```python
from build123d import *

# Parameters (mm, degrees)
SKETCH1_R           = 13.1
SKETCH1_R_2         = 1.75
BOSS_EXTRUDE1_DEPTH = 7
SKETCH2_R           = 13.1
SKETCH2_R_2         = 11
BOSS_EXTRUDE2_DEPTH = 2
SKETCH3_W           = 60
SKETCH3_H           = 16
SKETCH3_R           = 1.75
BOSS_EXTRUDE3_DEPTH = 4
SKETCH4_R           = 3.75
CUT_EXTRUDE1_DEPTH  = 4


with BuildPart() as part:
    # Sketch1 → Boss-Extrude1 (new body)
    with BuildSketch(Plane.XY):
        with BuildLine():
            Line((-30, -55), (30, -55))
            Line((30, -55), (30, -39))
            Line((30, -39), (24.811961667, 3.060483334))
            ThreePointArc((24.811961667, 3.060483334), (0, 25), (-24.811961667, 3.060483334))
            Line((-24.811961667, 3.060483334), (-30, -39))
            Line((-30, -39), (-30, -55))
        make_face()
        Circle(SKETCH1_R, mode=Mode.SUBTRACT)
        with Locations((-20, -47)):
            Circle(SKETCH1_R_2, mode=Mode.SUBTRACT)
        with Locations((20, -47)):
            Circle(SKETCH1_R_2, mode=Mode.SUBTRACT)
    extrude(amount=BOSS_EXTRUDE1_DEPTH)

    # Sketch2 → Boss-Extrude2 (add)
    with BuildSketch(Plane.XY.offset(7)):
        Circle(SKETCH2_R)
        Circle(SKETCH2_R_2, mode=Mode.SUBTRACT)
    extrude(amount=-BOSS_EXTRUDE2_DEPTH)

    # Sketch3 → Boss-Extrude3 (add)
    with BuildSketch(Plane.XY.offset(7)):
        with Locations((0, -47)):
            Rectangle(SKETCH3_W, SKETCH3_H)
        with Locations((20, -47)):
            Circle(SKETCH3_R, mode=Mode.SUBTRACT)
        with Locations((-20, -47)):
            Circle(SKETCH3_R, mode=Mode.SUBTRACT)
    extrude(amount=BOSS_EXTRUDE3_DEPTH)

    # Sketch4 → Cut-Extrude1 (cut)
    with BuildSketch(Plane(origin=(0, 0, 0), x_dir=(-1, 0, 0), z_dir=(0, 0, -1))):
        with Locations((-20, -47)):
            Circle(SKETCH4_R)
        with Locations((20, -47)):
            Circle(SKETCH4_R)
    extrude(amount=-CUT_EXTRUDE1_DEPTH, mode=Mode.SUBTRACT)


solid = part.part
```
Verification items for the finished model (mm, model axes). A direction names the side the tool comes from. Round coordinates to 2 decimals unless told otherwise and drop trailing zeros. Order: outer loops, then holes, each group sorted by start corner. A loop starts at its lowest first (then second) coordinate and runs counter-clockwise, first axis right, second up.
1) Draft check along X on faces 1 (the flat face through (30, -47, 5)), 2 (the flat face through (-21, -49, 4)), 3 (the flat face through (-27.37, -17.68, 3.45)). Enter one of: +X half, -X half, draft (parallel to the pull), parting line (faces both ways), or undercut.
Geometry says:
face 1: +X half
face 2: undercut
face 3: -X half
2) Cross-section at B-B, the plane x = 0. Record the cut outline in (y, z).
Geometry says:
outline: (-55, 0) - (-13.1, 0) - (-13.1, 5) - (-11, 5) - (-11, 7) - (-39, 7) - (-39, 11) - (-55, 11) - close; (11, 5) - (13.1, 5) - (13.1, 0) - (25, 0) - (25, 7) - (11, 7) - close
3) Cross-section at A-A, the plane z = 2.5. Record the cut outline in (x, y), plus the area to 3 significant figures.
Geometry says:
outline: (-30, -55) - (30, -55) - (30, -39) - (24.81, 3.06) arc R25 ccw to (-24.81, 3.06) - (-30, -39) - close; hole circle Ø7.5 at (-20, -47); hole circle Ø26.2 at (0, 0); hole circle Ø7.5 at (20, -47)
area: 3,470 mm2
4) Tool access check on faces 4 (the flat face through (0, -14, 7)), 5 (the flat face through (-30, -47, 5)), 6 (the flat face through (19, -49, 4)). Record the directions out of +Z, -Z, +X, -X, +Y, -Y that give a thin tool (end or side, any length) a straight path to the whole face; none if there is none.
Geometry says:
face 4: +Z, +X, -X, +Y
face 5: +Z, -Z, -X, +Y, -Y
face 6: -Z
5) Cross-section at C-C, the plane y = -47. Record the cut outline in (x, z), plus the area to 3 significant figures.
Geometry says:
outline: (-30, 0) - (-23.75, 0) - (-23.75, 4) - (-21.75, 4) - (-21.75, 11) - (-30, 11) - close; (-18.25, 4) - (-16.25, 4) - (-16.25, 0) - (16.25, 0) - (16.25, 4) - (18.25, 4) - (18.25, 11) - (-18.25, 11) - close; (21.75, 4) - (23.75, 4) - (23.75, 0) - (30, 0) - (30, 11) - (21.75, 11) - close
area: 551 mm2
6) Material ranges on line 1 (X direction, y = -47, z = 5.75); line 2 (Y direction, x = 20, z = 7.5); line 3 (Y direction, x = 0, z = 6.1), recorded low to high.
Geometry says:
line 1: x = -30 to -21.75, -18.25 to 18.25, 21.75 to 30
line 2: y = -55 to -48.75, -45.25 to -39
line 3: y = -55 to -11, 11 to 25
7) Cross-section at D-D, the plane z = 9. Record the cut outline in (x, y), plus the area to 3 significant figures.
Geometry says:
outline: (-30, -55) - (30, -55) - (30, -39) - (-30, -39) - close; hole circle Ø3.5 at (-20, -47); hole circle Ø3.5 at (20, -47)
area: 941 mm2
8) Depth check by flat-ended pin: pin 1 (8 mm diameter, centred on x = -3.5, y = 1, fed in from -Z); pin 2 (6 mm diameter, centred on x = 13, y = -27.5, fed in from -Z); pin 3 (4.5 mm diameter, centred on x = 20, y = -47, fed in from -Z); pin 4 (1 mm diameter, centred on x = -3.5, y = -35.5, fed in from +Z). Enter the tip coordinate at first touch or a pass-through.
Geometry says:
pin 1: passes through
pin 2: stops at z = 0
pin 3: stops at z = 4
pin 4: stops at z = 7
